Can you work these out from the model? Positions are in its coordinate system, mm. Face numbers are marked on the shaded views. Coordinates: 2 decimals unless noted, no trailing zeros. Order: outer loops, then holes, each group sorted by start corner. A loop starts at its lowest first (then second) coordinate and runs counter-clockwise, first axis right, second up. Notation, with made-up numbers: (4, -26) - (36, -26) arc R26 cw to (36, -9) - close; hole circle Ø9 at (26, 28). An arc over 180 degrees is marked (long way). Use a Markdown table: item, result. Add a question column.
(1) For pin 1 Ø3.5 at (x, z) = (31.82, 21.21) entering from +Y; pin 2 Ø1.5 at (x, y) = (-12.5, 2) entering from -Z; pin 3 Ø1.5 at (x, y) = (-28, 2.5) entering from -Z, each with a flat end and sliding along its axis, tell me the tip position at first contact or that it passes through.
(2) We'd pull the mould along Y, two halves only. Please class the marked faces 1 and 2: pulls with the +Y half, pulls with the -Y half, needs draft (parallel to the pull), parting line crosses it, or undercut.
(3) If I drill on L1, parallel to X at y = 1.3, z = -4.5; L2, parallel to X at y = 2.45, z = 6.5; L3, parallel to Z at x = 3, y = 1.6, over which ranges is the centre line in solid material (lowest first)? Write a range as [from, to].
(4) I want a section at B-B (y = 0.7). State how many separate pieces and enclosed holes the cut face has, and give its area (3 significant figures).
(5) I want a section at A-A (z = 7.5). List the corners of the cut face in (x, y) for me, and give its area (3 significant figures).
```python
from build123d import *

# Parameters (mm, degrees)
SKETCH_1_R          = 1.5
EXTRUDE_1_DEPTH     = 3
SKETCH_2_R          = 2.75
CUT_EXTRUDE_1_DEPTH = 1
SKETCH_3_R          = 1.5
SKETCH_3_W          = 24
SKETCH_3_H          = 6
SKETCH_3_W_2        = 6
SKETCH_3_H_2        = 18
CUT_EXTRUDE_2_DEPTH = 10
CUT_EXTRUDE_3_DEPTH = 10
EXTRUDE_2_DEPTH     = 3
CUT_EXTRUDE_4_DEPTH = 3
CUT_EXTRUDE_5_DEPTH = 10


with BuildPart() as part:
    # 草图1 → 凸台-拉伸1 (new body)
    with BuildSketch(Plane(origin=(0, 0, 0), x_dir=(1, 0, 0), z_dir=(0, 1, 0))):
        with BuildLine():
            Line((-10.325901808, 48), (10.325901808, 48))
            ThreePointArc((10.325901808, 48), (12.622002402, 47.543277195), (14.568542495, 46.242640687))
            Line((14.568542495, 46.242640687), (30.405591591, 30.405591591))
            ThreePointArc((30.405591591, 30.405591591), (33.396603497, 27.086285733), (36.027027027, 23.474524992))
            ThreePointArc((36.027027027, 23.474524992), (36.751615519, 21.907494269), (37, 20.199009877))
            Line((37, 20.199009877), (37, -20.199009877))
            ThreePointArc((37, -20.199009877), (36.751615519, -21.907494269), (36.027027027, -23.474524992))
            ThreePointArc((36.027027027, -23.474524992), (33.396603497, -27.086285733), (30.405591591, -30.405591591))
            Line((30.405591591, -30.405591591), (14.568542495, -46.242640687))
            ThreePointArc((14.568542495, -46.242640687), (12.622002402, -47.543277195), (10.325901808, -48))
            Line((10.325901808, -48), (-10.325901808, -48))
            ThreePointArc((-10.325901808, -48), (-12.622002402, -47.543277195), (-14.568542495, -46.242640687))
            Line((-14.568542495, -46.242640687), (-30.405591591, -30.405591591))
            ThreePointArc((-30.405591591, -30.405591591), (-33.396603497, -27.086285733), (-36.027027027, -23.474524992))
            ThreePointArc((-36.027027027, -23.474524992), (-36.751615519, -21.907494269), (-37, -20.199009877))
            Line((-37, -20.199009877), (-37, 20.199009877))
            ThreePointArc((-37, 20.199009877), (-36.751615519, 21.907494269), (-36.027027027, 23.474524992))
            ThreePointArc((-36.027027027, 23.474524992), (-33.396603497, 27.086285733), (-30.405591591, 30.405591591))
            Line((-30.405591591, 30.405591591), (-14.568542495, 46.242640687))
            ThreePointArc((-14.568542495, 46.242640687), (-12.622002402, 47.543277195), (-10.325901808, 48))
        make_face()
        with Locations(Location((-21.213203436, 31.819805153, 0), (0, 0, 270))):
            Circle(SKETCH_1_R, mode=Mode.SUBTRACT)
        with Locations(Location((-31.819805153, 21.213203436, 0), (0, 0, 270))):
            Circle(SKETCH_1_R, mode=Mode.SUBTRACT)
        with Locations(Location((31.819805153, 21.213203436, 0), (0, 0, 90))):
            Circle(SKETCH_1_R, mode=Mode.SUBTRACT)
        with Locations(Location((21.213203436, 31.819805153, 0), (0, 0, 90))):
            Circle(SKETCH_1_R, mode=Mode.SUBTRACT)
        with Locations(Location((-31.819805153, -21.213203436, 0), (0, 0, 90))):
            Circle(SKETCH_1_R, mode=Mode.SUBTRACT)
        with Locations(Location((-21.213203436, -31.819805153, 0), (0, 0, 90))):
            Circle(SKETCH_1_R, mode=Mode.SUBTRACT)
        with Locations(Location((31.819805153, -21.213203436, 0), (0, 0, 270))):
            Circle(SKETCH_1_R, mode=Mode.SUBTRACT)
        with Locations(Location((21.213203436, -31.819805153, 0), (0, 0, 270))):
            Circle(SKETCH_1_R, mode=Mode.SUBTRACT)
    extrude(amount=EXTRUDE_1_DEPTH)

    # 草图2 → 切除-拉伸1 (cut)
    with BuildSketch(Plane(origin=(0, 3, 0), x_dir=(1, 0, 0), z_dir=(0, 1, 0))):
        with Locations(Location((-21.213203436, 31.819805153, 0), (0, 0, 270))):
            Circle(SKETCH_2_R)
        with Locations(Location((-31.819805153, 21.213203436, 0), (0, 0, 270))):
            Circle(SKETCH_2_R)
        with Locations(Location((21.213203436, 31.819805153, 0), (0, 0, 270))):
            Circle(SKETCH_2_R)
        with Locations(Location((31.819805153, 21.213203436, 0), (0, 0, 270))):
            Circle(SKETCH_2_R)
        with Locations(Location((-31.819805153, -21.213203436, 0), (0, 0, 270))):
            Circle(SKETCH_2_R)
        with Locations(Location((-21.213203436, -31.819805153, 0), (0, 0, 270))):
            Circle(SKETCH_2_R)
        with Locations(Location((21.213203436, -31.819805153, 0), (0, 0, 270))):
            Circle(SKETCH_2_R)
        with Locations(Location((31.819805153, -21.213203436, 0), (0, 0, 270))):
            Circle(SKETCH_2_R)
    extrude(amount=-CUT_EXTRUDE_1_DEPTH, mode=Mode.SUBTRACT)

    # 草图3 → 切除-拉伸2 (cut)
    with BuildSketch(Plane(origin=(0, 3, 0), x_dir=(1, 0, 0), z_dir=(0, 1, 0))):
        with Locations(Location((-34, 12.5, 0), (0, 0, 270))):
            Circle(SKETCH_3_R)
        with Locations(Location((-34, -12.5, 0), (0, 0, 270))):
            Circle(SKETCH_3_R)
        with Locations(Location((34, 12.5, 0), (0, 0, 270))):
            Circle(SKETCH_3_R)
        with Locations(Location((34, -12.5, 0), (0, 0, 270))):
            Circle(SKETCH_3_R)
        with Locations((0, -40)):
            Rectangle(SKETCH_3_W, SKETCH_3_H)
        with Locations((0, 42)):
            Rectangle(SKETCH_3_W, SKETCH_3_H)
        with Locations((31, 0)):
            Rectangle(SKETCH_3_W_2, SKETCH_3_H_2)
        with Locations((-31, 0)):
            Rectangle(SKETCH_3_W_2, SKETCH_3_H_2)
    extrude(amount=-CUT_EXTRUDE_2_DEPTH, mode=Mode.SUBTRACT)

    # 草图4 → 切除-拉伸3 (cut)
    with BuildSketch(Plane.XZ):
        with BuildLine():
            Line((-12.325901808, 46), (12.325901808, 46))
            ThreePointArc((12.325901808, 46), (14.622002402, 45.543277195), (16.568542495, 44.242640687))
            Line((16.568542495, 44.242640687), (16.568542495, 49))
            Line((16.568542495, 49), (-16.568542495, 49))
            Line((-16.568542495, 49), (-16.568542495, 44.242640687))
            ThreePointArc((-16.568542495, 44.242640687), (-14.622002402, 45.543277195), (-12.325901808, 46))
        make_face()
    extrude(amount=-CUT_EXTRUDE_3_DEPTH, mode=Mode.SUBTRACT)

    # 草图5 → 凸台-拉伸2 (add)
    with BuildSketch(Plane.XZ):
        Polygon((-12, 37), (-12, 36), (12, 36), (12, 37), (13, 37), (13, 43), (12, 43), (12, 44), (-12, 44), (-12, 43), (-13, 43), (-13, 37), align=None)
        with BuildLine():
            Line((-10.3, 42.808101317), (-2.5, 41))
            Line((-2.5, 41), (2.5, 41))
            Line((2.5, 41), (10.3, 42.808101317))
            ThreePointArc((10.3, 42.808101317), (11.962490365, 40.08199487), (11.1, 37.007642751))
            Line((11.1, 37.007642751), (2.5, 39))
            Line((2.5, 39), (-2.5, 39))
            Line((-2.5, 39), (-11.1, 37.007642751))
            ThreePointArc((-11.1, 37.007642751), (-11.962490365, 40.08199487), (-10.3, 42.808101317))
        make_face(mode=Mode.SUBTRACT)
    extrude(amount=-EXTRUDE_2_DEPTH)

    # 草图6 → 切除-拉伸4 (cut)
    with BuildSketch(Plane.XZ):
        with BuildLine():
            Line((-21.75, 5), (-21.75, -5))
            ThreePointArc((-21.75, -5), (-22.5, -5.75), (-23.25, -5))
            Line((-23.25, -5), (-23.25, 5))
            ThreePointArc((-23.25, 5), (-22.5, 5.75), (-21.75, 5))
        make_face()
        with BuildLine():
            Line((-3, 30.25), (3, 30.25))
            ThreePointArc((3, 30.25), (3.75, 29.5), (3, 28.75))
            Line((3, 28.75), (-3, 28.75))
            ThreePointArc((-3, 28.75), (-3.75, 29.5), (-3, 30.25))
        make_face()
        with BuildLine():
            Line((-3, -30.25), (3, -30.25))
            ThreePointArc((3, -30.25), (3.75, -29.5), (3, -28.75))
            Line((3, -28.75), (-3, -28.75))
            ThreePointArc((-3, -28.75), (-3.75, -29.5), (-3, -30.25))
        make_face()
        with BuildLine():
            Line((21.75, 5), (21.75, -5))
            ThreePointArc((21.75, -5), (22.5, -5.75), (23.25, -5))
            Line((23.25, -5), (23.25, 5))
            ThreePointArc((23.25, 5), (22.5, 5.75), (21.75, 5))
        make_face()
    extrude(amount=-CUT_EXTRUDE_4_DEPTH, mode=Mode.SUBTRACT)

    # 草图7 → 切除-拉伸5 (cut)
    with BuildSketch(Plane.XZ):
        with BuildLine():
            Line((-20.39696962, 39), (-35.001785669, 24.395183951))
            Line((-35.001785669, 24.395183951), (-36.027027027, 23.474524992))
            Line((-36.027027027, 23.474524992), (-38.280094512, 25.727592477))
            Line((-38.280094512, 25.727592477), (-20.995221523, 43.012465466))
            Line((-20.995221523, 43.012465466), (-19.39696962, 41.414213562))
            ThreePointArc((-19.39696962, 41.414213562), (-20.137078087, 40.306562965), (-20.39696962, 39))
        make_face()
        with BuildLine():
            Line((38.280094512, 25.727592477), (36.027027027, 23.474524992))
            Line((36.027027027, 23.474524992), (35.001785669, 24.395183951))
            Line((35.001785669, 24.395183951), (20.39696962, 39))
            ThreePointArc((20.39696962, 39), (20.137078087, 40.306562965), (19.39696962, 41.414213562))
            Line((19.39696962, 41.414213562), (20.995221523, 43.012465466))
            Line((20.995221523, 43.012465466), (38.280094512, 25.727592477))
        make_face()
        with BuildLine():
            Line((35.001785669, -24.395183951), (36.027027027, -23.474524992))
            Line((36.027027027, -23.474524992), (38.280094512, -25.727592477))
            Line((38.280094512, -25.727592477), (20.995221523, -43.012465466))
            Line((20.995221523, -43.012465466), (19.39696962, -41.414213562))
            ThreePointArc((19.39696962, -41.414213562), (20.137078087, -40.306562965), (20.39696962, -39))
            Line((20.39696962, -39), (35.001785669, -24.395183951))
        make_face()
        with BuildLine():
            Line((-20.995221523, -43.012465466), (-38.280094512, -25.727592477))
            Line((-38.280094512, -25.727592477), (-36.027027027, -23.474524992))
            Line((-36.027027027, -23.474524992), (-35.001785669, -24.395183951))
            Line((-35.001785669, -24.395183951), (-20.39696962, -39))
            ThreePointArc((-20.39696962, -39), (-20.137078087, -40.306562965), (-19.39696962, -41.414213562))
            Line((-19.39696962, -41.414213562), (-20.995221523, -43.012465466))
        make_face()
    extrude(amount=-CUT_EXTRUDE_5_DEPTH, mode=Mode.SUBTRACT)


solid = part.part
```
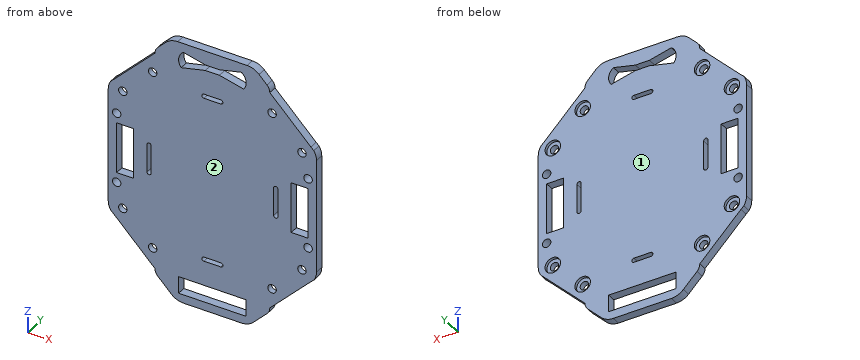
Answers follow:
| question | item | result |
|---|---|---|
| 1 | pin 1 | stops at y = 2 |
| 1 | pin 2 | stops at z = -47.83 |
| 1 | pin 3 | stops at z = -32.15 |
| 2 | face 1 | pulls with the +Y half |
| 2 | face 2 | pulls with the -Y half |
| 3 | L1 | x = [-37, -34], [-28, -23.25], [-21.75, 21.75], [23.25, 28], [34, 37] |
| 3 | L2 | x = [-37, -34], [-28, 28], [34, 37] |
| 3 | L3 | z = [-48, -45], [-39, -30.25], [-28.75, 28.75], [30.25, 38.88], [41.12, 46] |
| 4 | separate pieces | 1 |
| 4 | enclosed holes | 20 |
| 4 | area | 5,190 mm² |
| 5 | outline | (-37, 0) - (-34, 0) - (-34, 3) - (-37, 3) - close; (-28, 0) - (28, 0) - (28, 3) - (-28, 3) - close; (34, 0) - (37, 0) - (37, 3) - (34, 3) - close |
| 5 | area | 186 mm² |
